The listing builds one solid part. Answer for the finished solid, in the listing's coordinates (mm). Face numbers are marked on the shaded views. A direction names the side the tool comes from. Round coordinates to 2 decimals unless told otherwise and drop trailing zeros. Loops run counter-clockwise (first coordinate to the right, second up) from the corner with the lowest first, then second, coordinate; pieces in that order, holes last. Notation, with made-up numbers: (-20, 89.5) - (29, 89.5) arc R29 cw to (29, 126.5) - close; hole circle Ø5 at (16, 16). An arc over 180 degrees is marked (long way). One line per question, with ' | ' between items. Start each with the question number.
from build123d import *

# Parameters (mm, degrees)
SKETCH2_W           = 80
SKETCH2_H           = 30
SKETCH2_R           = 1.5
SKETCH2_R_2         = 3.4
BOSS_EXTRUDE1_DEPTH = 2
SKETCH3_W           = 6
SKETCH3_H           = 1.5
BOSS_EXTRUDE2_DEPTH = 13
SKETCH9_R           = 4
SKETCH9_R_2         = 1.5
BOSS_EXTRUDE4_DEPTH = 11
FILLET1_R           = 0.5
CHAMFER1_SIZE       = 2


with BuildPart() as part:
    # Sketch2 → Boss-Extrude1 (new body)
    with BuildSketch(Plane(origin=(0, 0, 0), x_dir=(1, 0, 0), z_dir=(0, 1, 0))):
        with Locations((25, 1)):
            Rectangle(SKETCH2_W, SKETCH2_H)
        with Locations(Location((0, 0, 0), (0, 0, 270))):  # turned: the seam where the file's is
            Circle(SKETCH2_R, mode=Mode.SUBTRACT)
        with Locations(Location((50, 0, 0), (0, 0, 270))):  # turned: the seam where the file's is
            Circle(SKETCH2_R, mode=Mode.SUBTRACT)
        with Locations(Location((25, 6, 0), (0, 0, 270))):  # turned: the seam where the file's is
            Circle(SKETCH2_R_2, mode=Mode.SUBTRACT)
    extrude(amount=BOSS_EXTRUDE1_DEPTH)

    # Sketch3 → Boss-Extrude2 (add)
    with BuildSketch(Plane(origin=(0, 2, 0), x_dir=(1, 0, 0), z_dir=(0, 1, 0))):
        Polygon((6, -14), (44, -14), (41, -12.5), (9, -12.5), align=None)
        with Locations((16.5, 15.25)):
            Rectangle(SKETCH3_W, SKETCH3_H)
        with Locations((33.5, 15.25)):
            Rectangle(SKETCH3_W, SKETCH3_H)
    extrude(amount=BOSS_EXTRUDE2_DEPTH)

    # Sketch9 → Boss-Extrude4 (add)
    with BuildSketch(Plane(origin=(0, 2, 0), x_dir=(1, 0, 0), z_dir=(0, 1, 0))):
        with Locations(Location((50, 0, 0), (0, 0, 90))):  # turned: the seam where the file's is
            Circle(SKETCH9_R)
        with Locations(Location((50, 0, 0), (0, 0, 270))):  # turned: the seam where the file's is
            Circle(SKETCH9_R_2, mode=Mode.SUBTRACT)
        with Locations(Location((0, 0, 0), (0, 0, 90))):  # turned: the seam where the file's is
            Circle(SKETCH9_R)
        with Locations(Location((0, 0, 0), (0, 0, 270))):  # turned: the seam where the file's is
            Circle(SKETCH9_R_2, mode=Mode.SUBTRACT)
    extrude(amount=BOSS_EXTRUDE4_DEPTH)

    # Fillet1
    fillet1_edges = [part.edges().sort_by_distance(p)[0] for p in [
        (6, 8.5, 14),
        (44, 8.5, 14),
    ]]
    fillet(fillet1_edges, radius=FILLET1_R)

    # Chamfer1
    chamfer1_edges = [part.edges().sort_by_distance(p)[0] for p in [
        (25, 2, 12.5),
    ]]
    chamfer(chamfer1_edges, length=CHAMFER1_SIZE)


solid = part.part
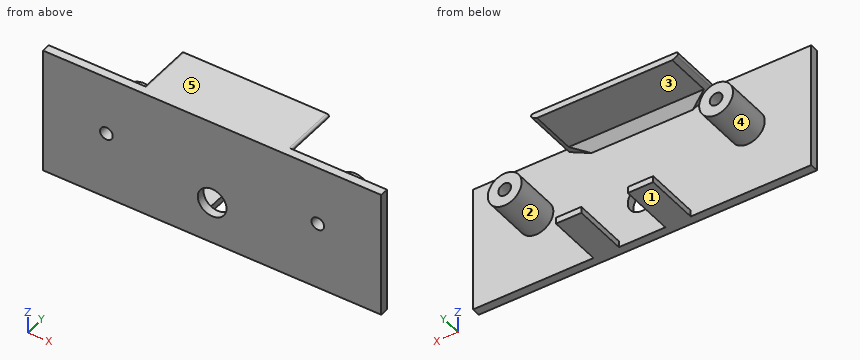
(1) Find section A-A on x = 25. Write down the section's boundary in (y, z), plus the area to 3 significant figures.
(2) A tool of negligible diameter and unlimited length cuts with its end or side. For the marked faces 3, 4 and 5, from which of +Z, -Z, +X, -X, +Y, -Y can it reach the whole face along a straight path? Write none if from no direction.
(3) Each of these flat-tipped pins is pushed along its axis until it touches: P1, Ø3, axis at y = 11.5, z = 1.5, coming from the +X side; P2, Ø1.2, axis at y = 7.5, z = -15.5, coming from the +X side; P3, Ø5.5, axis at x = 25.5, y = 8, coming from the -Z side; P4, Ø8, axis at x = 36.5, z = -4, coming from the -Y side. Where does it stop, or does it pass through?
(4) Determine the mould class of the marked faces 1 and 2 for opening direction X: pulls with the +X half, pulls with the -X half, needs draft (parallel to the pull), parting line crosses it, or undercut.
(5) Find section B-B on y = 10.5. Write down the section's boundary in (x, z), plus the area to 3 significant figures.
(6) Consider L1, parallel to X at y = 10, z = 0; L2, parallel to Z at x = 31, y = 5; L3, parallel to Y at x = -1, z = 6.75. Determine where each line is inside the solid, lowest interval first.
(7) Find section C-C on z = -6. Write down the section's boundary in (x, y), plus the area to 3 significant figures.
(8) Find section D-D on y = 1. Write down the section's boundary in (x, z), plus the area to 3 significant figures.
Answer below:
1) outline: (0, -16) - (2, -16) - (2, -9.4) - (0, -9.4) - close; (0, -2.6) - (2, -2.6) - (2, 10.5) - (4, 12.5) - (15, 12.5) - (15, 14) - (0, 14) - close | area: 67.9 mm2
2) face 3: +X, -X, +Y | face 4: +Y | face 5: +Z, +X, -X, +Y, -Y
3) P1: x = 54 | P2: x = 36.5 | P3: z = 12.5 | P4: y = 0
4) face 1: needs draft | face 2: undercut
5) outline: circle Ø8 at (0, 0); (7.89, 13.05) - (9, 12.5) - (41, 12.5) - (42.11, 13.05) arc R0.5 ccw to (41.88, 14) - (8.12, 14) arc R0.5 ccw to start; (13.5, -16) - (19.5, -16) - (19.5, -14.5) - (13.5, -14.5) - close; (30.5, -16) - (36.5, -16) - (36.5, -14.5) - (30.5, -14.5) - close; circle Ø8 at (50, 0); hole circle Ø3 at (0, 0); hole circle Ø3 at (50, 0) | area: 155 mm2
6) L1: -4 to -1.5, 1.5 to 4, 46 to 48.5, 51.5 to 54 | L2: -16 to -14.5, 12.5 to 14 | L3: 0 to 2
7) outline: (-15, 0) - (21.6, 0) - (21.6, 2) - (-15, 2) - close; (28.4, 0) - (65, 0) - (65, 2) - (28.4, 2) - close | area: 146 mm2
8) outline: (-15, -16) - (65, -16) - (65, 14) - (-15, 14) - close; hole circle Ø3 at (0, 0); hole circle Ø6.8 at (25, -6); hole circle Ø3 at (50, 0) | area: 2,350 mm2
